```python
from build123d import *

# Parameters (mm, degrees)
BOSS_EXTRUDE1_DEPTH = 152.4
SKETCH2_R           = 2.5796875
CUT_EXTRUDE1_DEPTH  = 2.5875


with BuildPart() as part:
    # Sketch1 → Boss-Extrude1 (new body)
    with BuildSketch(Plane.XY):
        Polygon((-6.35, 19.05), (-4.7625, 19.05), (-4.7625, 15.875), (-1.5875, 15.875), (-1.5875, 19.05), (0, 19.05), (0, 0), (-1.5875, 0), (-1.5875, 14.2875), (-6.35, 14.2875), align=None)
    extrude(amount=BOSS_EXTRUDE1_DEPTH)

    # Sketch2 → Cut-Extrude1 (cut, through all)
    with BuildSketch(Plane.ZY.offset(1.5875)):
        with Locations((12.7, 7.9375)):
            Circle(SKETCH2_R)
        with Locations((139.7, 7.9375)):
            Circle(SKETCH2_R)
    extrude(amount=-CUT_EXTRUDE1_DEPTH, mode=Mode.SUBTRACT)


solid = part.part
```
The listing builds one solid part. Answer for the finished solid, in the listing's coordinates (mm). A direction names the side the tool comes from. Round coordinates to 2 decimals unless told otherwise and drop trailing zeros.
1) Given P1, Ø4, axis at y = 10, z = 78, coming from the -X side, flat-ended and moving along its own axis, determine where the tip first touches the part or whether it passes through.
Outcome:
P1: stops at x = -1.59
2) Consider line 1 (X direction, y = 16.75, z = 100); line 2 (Y direction, x = -0.5, z = 139.7); line 3 (Z direction, x = -1.25, y = 7.5). Determine where each line is inside the solid, lowest interval first.
Outcome:
line 1: x = -6.35 to -4.76, -1.59 to 0
line 2: y = 0 to 5.36, 10.52 to 19.05
line 3: z = 0 to 10.16, 15.24 to 137.16, 142.24 to 152.4
3) For a pull along Z with two mould halves and no side action, classify faces 1 (the face through (-0.8, 8.71, 142.16)), 2 (the face through (-4.762, 17, 75)), 3 (the face through (-1, 11, 152.4)) as released by +Z, released by -Z, zero draft, split by the parting line, or undercut.
Outcome:
face 1: undercut
face 2: zero draft
face 3: released by +Z
4) For faces 4 (the face through (0, 10, 75)), 5 (the face through (-1.588, 7, 75)), 6 (the face through (-3, 15.875, 75)), determine the directions among +Z, -Z, +X, -X, +Y, -Y from which every point of the face is accessible in a straight line to the end or side of a thin tool.
Outcome:
face 4: +Z, -Z, +X, +Y, -Y
face 5: +Z, -Z, -X, -Y
face 6: +Z, -Z, +Y
